Design review of the part built by this model. Coordinates are the model's own, in mm. Face numbers are marked on the shaded views. A direction names the side the tool comes from. Round coordinates to 2 decimals unless told otherwise and drop trailing zeros. Loops run counter-clockwise (first coordinate to the right, second up) from the corner with the lowest first, then second, coordinate; pieces in that order, holes last. Notation, with made-up numbers: (79, 48) - (131, 48) arc R9 cw to (131, 57) - close; hole circle Ø2 at (55.25, 77.25). An arc over 180 degrees is marked (long way). Use one line per item in the form item = value. Start each with the question number.
(1) We need section A-A, the plane z = 0.3. Write out the cut boundary in (x, y) (3 decimals), then the cut area to 3 significant figures.
(2) We need section B-B, the plane x = -1.75. Write out the cut boundary in (y, z), then the cut area to 3 significant figures.
(3) We need section C-C, the plane y = 0. Write out the cut boundary in (x, z) (3 decimals).
(4) Wall thickness on probe 1 along X at (y, z) = (-1.4, 0.6); probe 2 along X at (y, z) = (2.8, 0.95); probe 3 along Y at (x, z) = (-2, 0.1): over which ranges is each line inside the solid? List them lowest first. Write a range as [from, to].
(5) The part is to be moulded in two halves that separate along Y. For the marked faces 1, 2, 3 and 4, say which applies: released by +Y, released by -Y, zero draft, split by the parting line, or undercut.
(6) We need section D-D, the plane y = 1.4. Write out the cut boundary in (x, z).
(7) Machinability: for the marked faces 5, 6, 7 and 8, which of the approach directions +Z, -Z, +X, -X, +Y, -Y give a long, thin tool a straight path to every point of the face, cutting with its end or side? Answer none if there is none.
from build123d import *

# Parameters (mm, degrees)
BOSS_EXTRU_1_DEPTH      = 1
ESQUISSE4_R             = 0.125
ENL_V_MAT_EXTRU_1_DEPTH = 2


with BuildPart() as part:
    # Esquisse3 → Boss.-Extru.1 (new body)
    with BuildSketch(Plane.XY):
        Polygon((0, 3.217227712), (0.720420955, 1), (3.051752136, 1), (1.165665591, -0.370322087), (1.886086545, -2.587549798), (0, -1.217227712), (-1.886086545, -2.587549798), (-1.165665591, -0.370322087), (-3.051752136, 1), (-0.720420955, 1), align=None)
    extrude(amount=BOSS_EXTRU_1_DEPTH)

    # Esquisse4 → Enlèv. mat.-Extru.1 (cut, through all)
    with BuildSketch(Plane(origin=(0, 0, 0), x_dir=(-1, 0, 0), z_dir=(0, 0, -1))):
        Circle(ESQUISSE4_R)
    extrude(amount=-ENL_V_MAT_EXTRU_1_DEPTH, mode=Mode.SUBTRACT)


solid = part.part
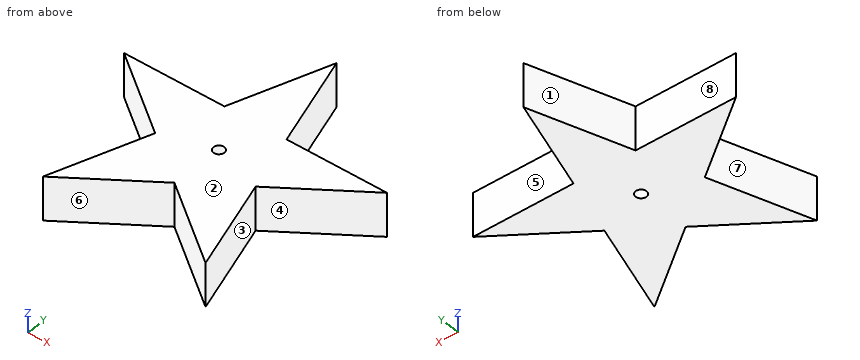
Data:
q1.outline = (-3.052, 1) - (-1.166, -0.37) - (-1.886, -2.588) - (0, -1.217) - (1.886, -2.588) - (1.166, -0.37) - (3.052, 1) - (0.72, 1) - (0, 3.217) - (-0.72, 1) - close; hole circle Ø0.25 at (0, 0)
q1.area = 11.5 mm^2
q2.outline = (-2.49, 0) - (-2.17, 0) - (-2.17, 1) - (-2.49, 1) - close; (0.05, 0) - (1, 0) - (1, 1) - (0.05, 1) - close
q2.area = 1.27 mm^2
q3.outline = (-1.675, 0) - (-0.125, 0) - (-0.125, 1) - (-1.675, 1) - close; (0.125, 0) - (1.675, 0) - (1.675, 1) - (0.125, 1) - close
q4.probe_1 = [-1.5, -0.25], [0.25, 1.5]
q4.probe_2 = [-0.14, 0.14]
q4.probe_3 = [0.24, 1]
q5.face_1 = released by +Y
q5.face_2 = zero draft
q5.face_3 = undercut
q5.face_4 = undercut
q6.outline = (-0.59, 0) - (0.59, 0) - (0.59, 1) - (-0.59, 1) - close
q7.face_5 = +Z, -Z, +X, +Y
q7.face_6 = +Z, -Z, -Y
q7.face_7 = +Z, -Z, -X
q7.face_8 = +Z, -Z, -X, +Y
